Check sheet for the drawn part. Datum: minimum x, y, z corner. Units: mm. A direction names the side the tool comes from. Coordinates: 2 decimals unless noted, no trailing zeros. Write item = value, one per line. Start each with the question number.
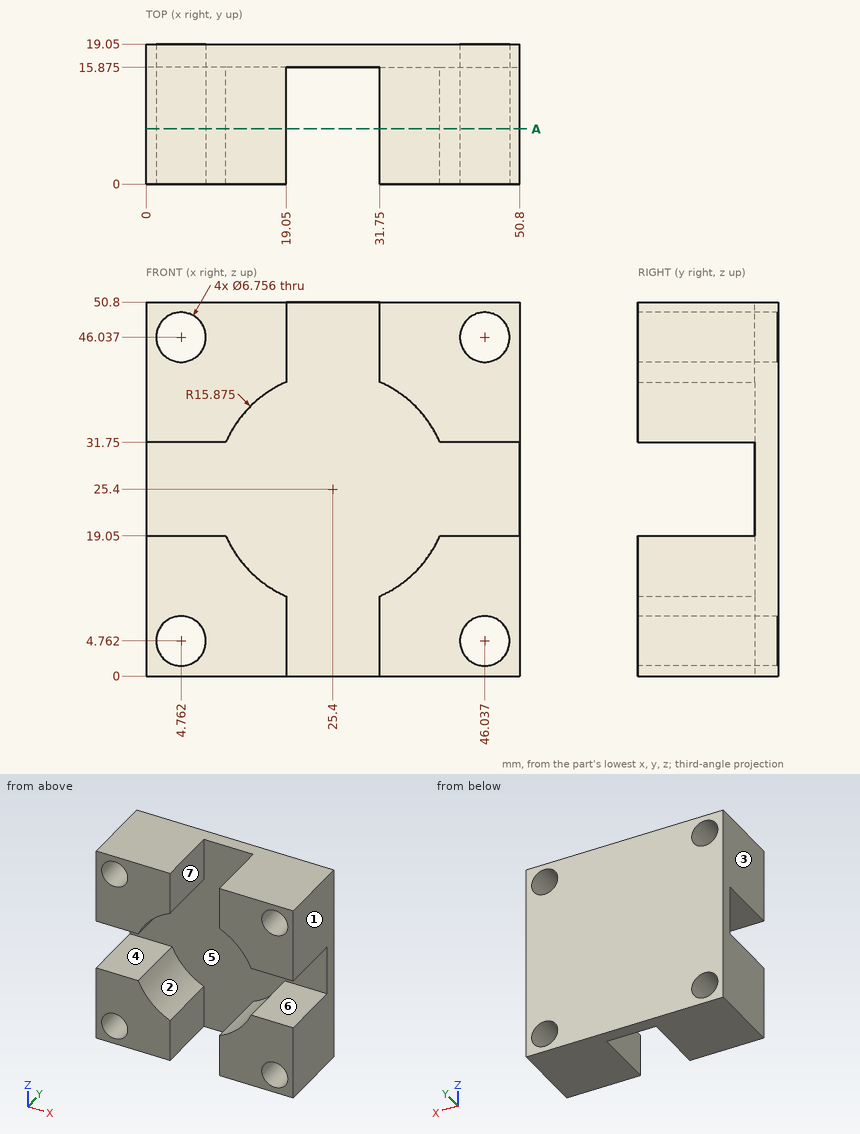
Item 1: Mould release check, pull along X, two halves, no side actions. Record for the marked faces 1, 2, 3 and 4: pulls with the +X half, pulls with the -X half, needs draft (parallel to the pull), parting line crosses it, or undercut.
Item 2: Section check A-A (y = 7.5). State how many separate pieces and enclosed holes the cut face has, then the cut area to 3 significant figures.
Item 3: Tool access check on the marked faces 5, 6 and 7. Record the directions out of +Z, -Z, +X, -X, +Y, -Y that give a thin tool (end or side, any length) a straight path to the whole face; none if there is none.
Item 4: Thickness scan on line 1 (Z direction, x = 46.5, y = 16.5) (1 decimal); line 2 (X direction, y = 16.75, z = 44) (1 decimal); line 3 (Z direction, x = 9, y = 10.5). Record the ranges inside material, lowest first.
Item 5: Gauge pin test, flat end, axial feed: P1, Ø4, axis at x = 36.5, y = 11.5, coming from the -Z side. Record the tip position at first contact, or that the pin passes through.
Filled sheet:
q1.face_1 = pulls with the +X half
q1.face_2 = undercut
q1.face_3 = pulls with the -X half
q1.face_4 = needs draft
q2.separate_pieces = 4
q2.enclosed_holes = 4
q2.area = 1,140 mm^2
q3.face_5 = -Y
q3.face_6 = +X, -X, -Y
q3.face_7 = +Z, -Z, -Y
q4.line_1 = 0 to 1.4, 8.1 to 42.7, 49.4 to 50.8
q4.line_2 = 0 to 2.1, 7.5 to 43.3, 48.7 to 50.8
q4.line_3 = 0 to 19.05, 31.75 to 50.8
q5.P1 = 0
